Can you work these out from the drawing? Everything is in mm from the part's minimum corner. A direction names the side the tool comes from. Give positions to 0.01 mm unless a question says otherwise; leave off trailing zeros. Write each loop counter-clockwise with the first axis right and the second up, starting at its lowest first coordinate (ties: lowest second). Pieces come first, ordered by that corner, then holes. Notation, with made-up numbers: (86, -4.5) -> (120, -4.5) arc R20 ccw to (120, 34.5) -> close; hole circle Ø7 at (43.5, 31). An arc over 180 degrees is marked (long way). Use one line per item in the form item = value.
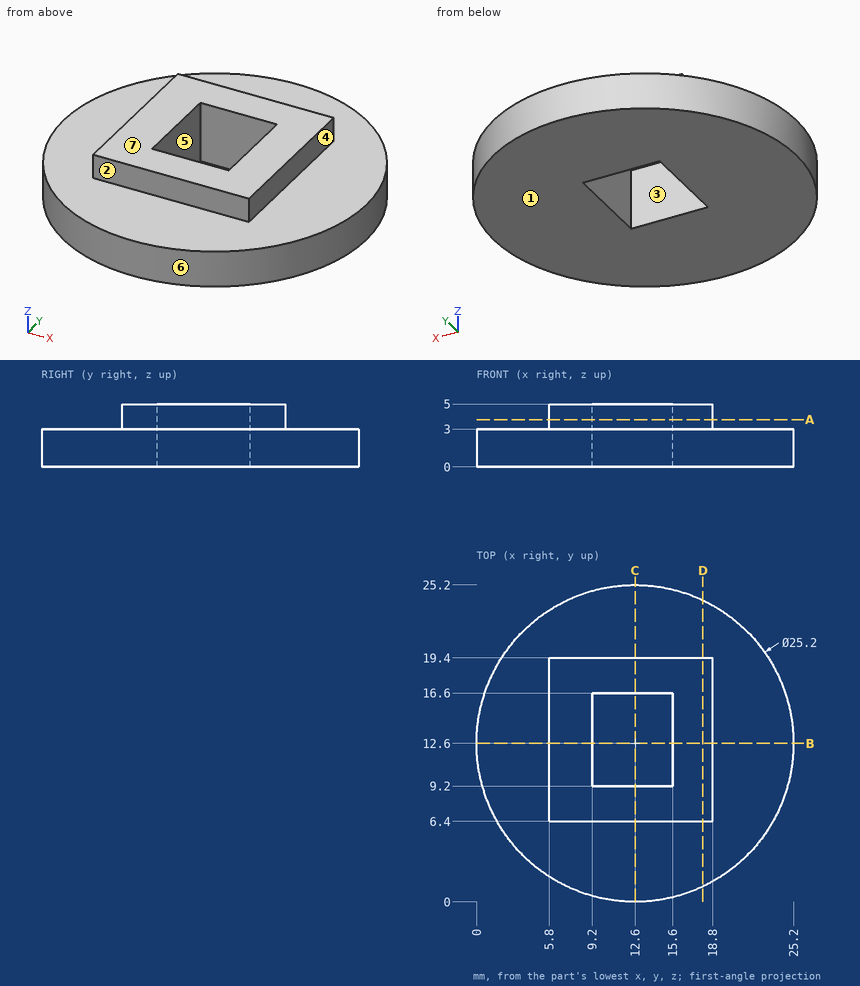
Q1. I want a section at C-C, the plane x = 12.6. Write out the boundary of the cut face in (y, z), and give its area (3 significant figures).
Result set:
outline = (0, 0) -> (9.2, 0) -> (9.2, 5) -> (6.4, 5) -> (6.4, 3) -> (0, 3) -> close; (16.6, 0) -> (25.2, 0) -> (25.2, 3) -> (19.4, 3) -> (19.4, 5) -> (16.6, 5) -> close
area = 64.6 mm2
Q2. Will these pins go through, and if not, where does the flat tip stop? pin 1 Ø1.5 at (y, z) = (9.5, 3.5) entering from +X; pin 2 Ø1 at (x, z) = (14, 4.5) entering from -Y; pin 3 Ø2.5 at (y, z) = (11.5, 3.5) entering from +X; pin 4 Ø1 at (y, z) = (11, 4) entering from -X.
Result set:
pin_1 = 24.94
pin_2 = 6.4
pin_3 = 25.2
pin_4 = 5.8
Q3. If I drill on line 1 along X through (y, z) = (16, 4.1); line 2 along Y through (x, z) = (9.5, 3.1); line 3 along X through (y, z) = (17.5, 3.6), over which ranges is the centre line in solid material (lowest first)? Write a range as from..to.
Result set:
line_1 = 5.8..9.2, 15.6..18.8
line_2 = 6.4..9.2, 16.6..19.4
line_3 = 5.8..18.8
Q4. If we mould it in two halves opening along X, with no side actions, what happens to the marked faces 4, 5, 6 and 7? For each: +X half, -X half, draft (parallel to the pull), parting line (faces both ways), or undercut.
Result set:
face_4 = +X half
face_5 = undercut
face_6 = parting line
face_7 = draft
Q5. I want a section at A-A, the plane z = 3.75. Write out the boundary of the cut face in (x, y), and give its area (3 significant figures).
Result set:
outline = (5.8, 6.4) -> (18.8, 6.4) -> (18.8, 19.4) -> (5.8, 19.4) -> close; hole (9.2, 9.2) -> (15.6, 9.2) -> (15.6, 16.6) -> (9.2, 16.6) -> close
area = 122 mm2
Q6. Which directions (+Z, -Z, +X, -X, +Y, -Y) give clear straight access to the entire face, cutting with the end or side of a thin tool? Please do the marked faces 1, 2 and 3.
Result set:
face_1 = -Z, +X, -X, +Y, -Y
face_2 = +Z, +X, -X, -Y
face_3 = +Z, -Z
Q7. I want a section at D-D, the plane x = 18. Write out the boundary of the cut face in (y, z).
Result set:
outline = (1.22, 0) -> (23.98, 0) -> (23.98, 3) -> (19.4, 3) -> (19.4, 5) -> (6.4, 5) -> (6.4, 3) -> (1.22, 3) -> close
Q8. I want a section at B-B, the plane y = 12.6. Write out the boundary of the cut face in (x, z), and give its area (3 significant figures).
Result set:
outline = (0, 0) -> (9.2, 0) -> (9.2, 5) -> (5.8, 5) -> (5.8, 3) -> (0, 3) -> close; (15.6, 0) -> (25.2, 0) -> (25.2, 3) -> (18.8, 3) -> (18.8, 5) -> (15.6, 5) -> close
area = 69.6 mm2
